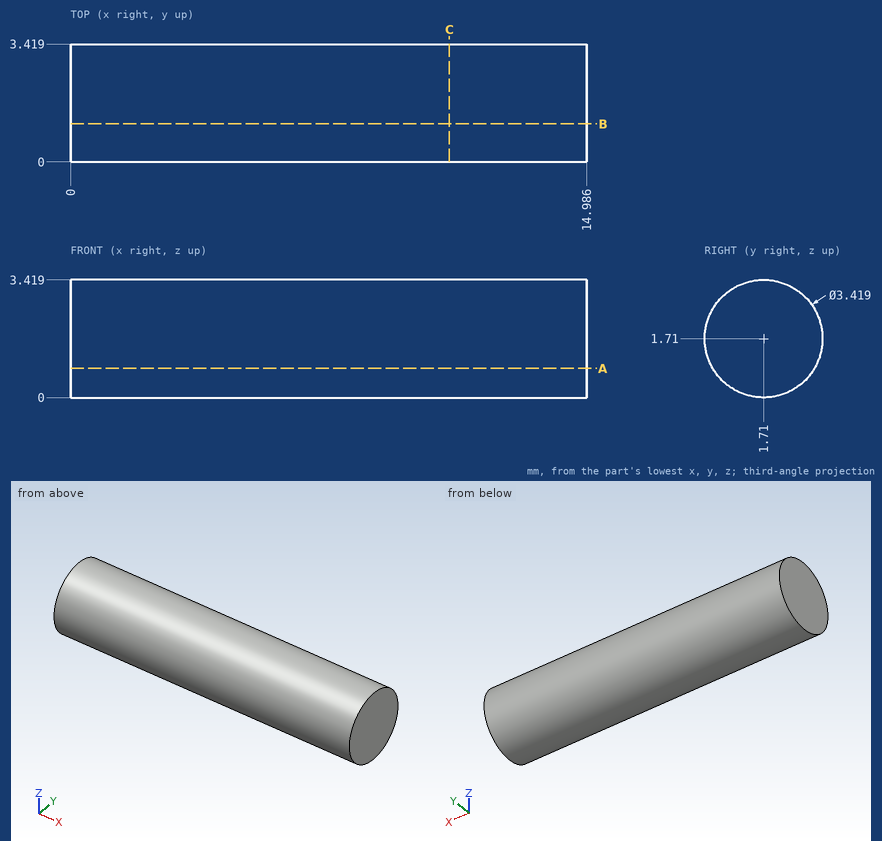
Study the drawing (mm; zero at the part's minimum x, y, z) and answer. Coordinates: 2 decimals unless noted, no trailing zeros. Write each loop counter-clockwise with the first axis right and the second up, starting at its lowest first coordinate (ties: lowest second). Pieces come first, ordered by that corner, then holes. Notation, with made-up numbers: (-38, -36.75) - (-10, -36.75) arc R21 ccw to (-10, -3.75) - close; hole circle Ø7 at (2, -27.75). An arc over 180 degrees is marked (long way). One line per item, written item: value.
1) Find section A-A (z = 0.85). Give the vertices of the cut face in (x, y) (1 decimal).
Geometry check:
outline: (0, 0.2) - (15, 0.2) - (15, 3.2) - (0, 3.2) - close
2) Consider line 1 along Z through (x, y) = (4.75, 1.65); line 2 along Y through (x, z) = (3.25, 1.6) (1 decimal); line 3 along Z through (x, y) = (1.5, 0.5) (1 decimal). Determine where each line is inside the solid, lowest interval first. Write a range as from..to.
Geometry check:
line 1: z = 0..3.42
line 2: y = 0..3.4
line 3: z = 0.5..2.9
3) Find section C-C (x = 11). Give the vertices of the cut face in (y, z).
Geometry check:
outline: circle Ø3.42 at (1.71, 1.71)
4) Find section B-B (y = 1.1). Give the vertices of the cut face in (x, z) (1 decimal).
Geometry check:
outline: (0, 0.1) - (15, 0.1) - (15, 3.3) - (0, 3.3) - close
